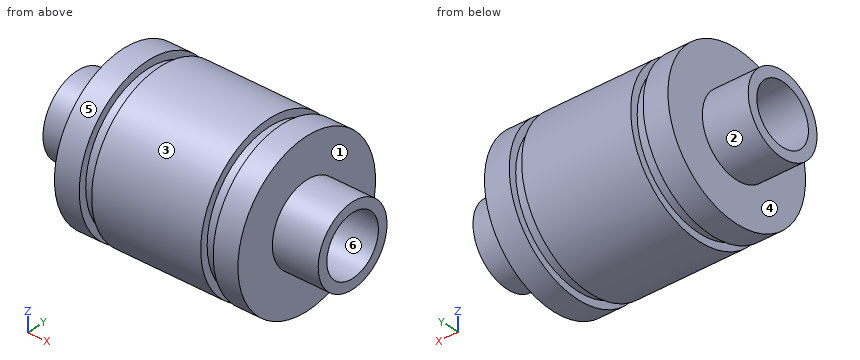
```python
from build123d import *

# Parameters (mm, degrees)
CROQUIS3_R            = 6
CORTAR_EXTRUIR1_DEPTH = 60.935381871


with BuildPart() as part:
    # Croquis2 → Revolución1 (revolve)
    with BuildSketch(Plane.XY, mode=Mode.PRIVATE) as revoluci_n1_sk:
        Polygon((0, 0), (18.5, 0), (27.75, 0), (27.75, 8), (18.5, 8), (18.5, 16), (13.5, 16), (13.5, 14.5), (11, 14.5), (11, 16), (-11, 16), (-11, 14.5), (-13.5, 14.5), (-13.5, 16), (-18.5, 16), (-18.5, 8), (-27.75, 8), (-27.75, 0), (-12.75, 0), align=None)
    revolve(revoluci_n1_sk.sketch.rotate(Axis((-12.75, 0, 0), (1, 0, 0)), 90), axis=Axis((-12.75, 0, 0), (1, 0, 0)))

    # Croquis3 → Cortar-Extruir1 (cut, through all)
    with BuildSketch(Plane.ZY.offset(27.75)):
        Circle(CROQUIS3_R)
    extrude(amount=-CORTAR_EXTRUIR1_DEPTH, mode=Mode.SUBTRACT)


solid = part.part
```
CAD build for the part. Positions are in the model's coordinates, mm. Face numbers are marked on the shaded views. A direction names the side the tool comes from. Round coordinates to 2 decimals unless told otherwise and drop trailing zeros. Order: outer loops, then holes, each group sorted by start corner. A loop starts at its lowest first (then second) coordinate and runs counter-clockwise, first axis right, second up. Notation, with made-up numbers: (8.5, 57) - (60.5, 57) arc R18 ccw to (60.5, 87) - close; hole circle Ø5 at (29.25, 44.25). An arc over 180 degrees is marked (long way). Use CSV: the item, a comma, the result in double quotes. Start each with the question number.
1) Wall check: L1, parallel to X at y = -9, z = 11.5; L2, parallel to Y at x = -2, z = 0; L3, parallel to X at y = 6, z = 7.5. Give the ranges that are in metal, low to high. Write a range as [from, to].
2) Tool access for the marked faces 1, 2 and 3: list every direction of +Z, -Z, +X, -X, +Y, -Y with a clear straight run to the whole face (end or side of a thin tool).
3) Saw through at C-C (x = 22). List the corners of the cut face in (y, z), and give its area (3 significant figures).
4) Saw through at D-D (z = 7). List the corners of the cut face in (x, y).
5) Two-plate mould, pull along Z, no slides. Class the marked faces 4, 5 and 6: pulls with the +Z half, pulls with the -Z half, needs draft (parallel to the pull), parting line crosses it, or undercut.
6) Pin check, flat tips, straight feed: pin 1 Ø2 at (x, y) = (21.5, -10) entering from +Z; pin 2 Ø1.5 at (y, z) = (-4.5, -8) entering from +X; pin 3 Ø4 at (y, z) = (-2, -10) entering from -X; pin 4 Ø8 at (x, z) = (-3.5, 8) entering from +Y. Stop position of each tip, or through.
Values follow:
1,L1,"x = [-18.5, -13.5], [-11, 11], [13.5, 18.5]"
1,L2,"y = [-16, -6], [6, 16]"
1,L3,"x = [-18.5, 18.5]"
2,face 1,"+X"
2,face 2,"-X"
2,face 3,"+X, -X"
3,outline,"circle Ø16 at (0, 0); hole circle Ø12 at (0, 0)"
3,area,"88.0 mm2"
4,outline,"(-27.75, -3.87) - (-18.5, -3.87) - (-18.5, -14.39) - (-13.5, -14.39) - (-13.5, -12.7) - (-11, -12.7) - (-11, -14.39) - (11, -14.39) - (11, -12.7) - (13.5, -12.7) - (13.5, -14.39) - (18.5, -14.39) - (18.5, -3.87) - (27.75, -3.87) - (27.75, 3.87) - (18.5, 3.87) - (18.5, 14.39) - (13.5, 14.39) - (13.5, 12.7) - (11, 12.7) - (11, 14.39) - (-11, 14.39) - (-11, 12.7) - (-13.5, 12.7) - (-13.5, 14.39) - (-18.5, 14.39) - (-18.5, 3.87) - (-27.75, 3.87) - close"
5,face 4,"needs draft"
5,face 5,"parting line crosses it"
5,face 6,"undercut"
6,pin 1,"passes through"
6,pin 2,"stops at x = 18.5"
6,pin 3,"stops at x = -18.5"
6,pin 4,"stops at y = 15.49"
